Source: CAD feature listing. Evaluate the final solid. Frame: model axes, mm. A direction names the side the tool comes from. Coordinates: 2 decimals unless noted, no trailing zeros. Order: outer loops, then holes, each group sorted by start corner. A loop starts at its lowest first (then second) coordinate and runs counter-clockwise, first axis right, second up. Notation, with made-up numbers: (32.5, -33.5) - (78.5, -33.5) arc R25 cw to (78.5, -19.5) - close; hole circle Ø11 at (68.5, -31.5). An arc over 180 degrees is marked (long way). One line per question, with ' | ' between items. Start each with the question number.
(1) Line query: line 1 along Y through (x, z) = (3.5, 0.6); line 2 along X through (y, z) = (-6.75, 1.05); line 3 along Z through (x, y) = (18.25, -12.5). Output: solid intervals per line, ascending.
(2) Section A-A (z = 0.6). Return the cut outline in (x, y), then the cut area to 3 significant figures.
(3) Section B-B (y = -1.75). Return the cut outline in (x, z), then the cut area to 3 significant figures.
(4) Contact query for flat-ended pins moving along their axis: P1, Ø0.8, axis at x = 12.5, z = 1.5, coming from the -Y side; P2, Ø2.5, axis at x = 3.5, y = -2.1, coming from the +Z side; P3, Ø0.8, axis at x = 17, z = 1.5, coming from the +Y side. Output: stop coordinate, or through.
(5) Section D-D (y = -7.9). Return the cut outline in (x, z).
(6) Section C-C (x = 12.75). Return the cut outline in (y, z).
(7) Access query for faces 1 (the flat face through (14.035, -2, 1.5)), 2 (the flat face through (23.3, -0.5, 0.5)). Directions: +Z, -Z, +X, -X, +Y, -Y. A direction counts if a zero-diameter tool reaches every point of the face in a straight line with its end or side. Return the directions, or none.
(8) Draft query along Y for faces 3 (the cylindrical face through (22.5, -7.9, 0.5)), 4 (the cylindrical face through (22.5, -3.9, 0.5)), 5 (the flat face through (12, -2, 2)), 6 (the flat face through (11.8, -13.7, 0.5)). Return one class per face: +Y half, -Y half, draft (parallel to the pull), parting line (faces both ways), or undercut.
from build123d import *
from build123d.topology import SkipClean

# Parameters (mm, degrees)
SKETCH1_R           = 0.911145061
BOSS_EXTRUDE1_DEPTH = 1
SKETCH2_W           = 7.631466846
SKETCH2_H           = 13.7
BOSS_EXTRUDE2_DEPTH = 0.1
SKETCH3_W           = 5.617836281
SKETCH3_H           = 5.617836281
SKETCH3_W_2         = 4.333759416
SKETCH3_H_2         = 2.636943561
BOSS_EXTRUDE3_DEPTH = 2


with BuildPart() as part:
    # Sketch1 → Boss-Extrude1 (new body)
    with BuildSketch(Plane.XY):
        with BuildLine():
            Line((23.3, -2.7), (23.3, -3.1))
            ThreePointArc((23.3, -3.1), (22.5, -3.9), (23.3, -4.7))
            Line((23.3, -4.7), (23.3, -5.1))
            ThreePointArc((23.3, -5.1), (22.5, -5.9), (23.3, -6.7))
            Line((23.3, -6.7), (23.3, -7.1))
            ThreePointArc((23.3, -7.1), (22.5, -7.9), (23.3, -8.7))
            Line((23.3, -8.7), (23.3, -9.1))
            ThreePointArc((23.3, -9.1), (22.5, -9.9), (23.3, -10.7))
            Line((23.3, -10.7), (23.3, -11.1))
            ThreePointArc((23.3, -11.1), (22.5, -11.9), (23.3, -12.7))
            Line((23.3, -12.7), (23.3, -13.7))
            Line((23.3, -13.7), (0, -13.7))
            Line((0, -13.7), (0, 0))
            Line((0, 0), (23.3, 0))
            Line((23.3, 0), (23.3, -1.1))
            ThreePointArc((23.3, -1.1), (22.5, -1.9), (23.3, -2.7))
        make_face()
        with Locations((3.5, -2.1)):
            Circle(SKETCH1_R, mode=Mode.SUBTRACT)
    extrude(amount=BOSS_EXTRUDE1_DEPTH)

    # Sketch2 → Boss-Extrude2 (add)
    with SkipClean():  # the faces are left unmerged after this step: merging them gives an invalid solid
        with BuildSketch(Plane.XY.offset(1)):
            with Locations((3.815733423, -6.85)):
                Rectangle(SKETCH2_W, SKETCH2_H)
            with BuildLine():
                ThreePointArc((2.952848723, -2.828567637), (3.092783142, -1.284917334), (4.411145061, -2.1))
                ThreePointArc((4.411145061, -2.1), (3.907216858, -2.915082666), (2.952848723, -2.828567637))
            make_face(mode=Mode.SUBTRACT)
        extrude(amount=BOSS_EXTRUDE2_DEPTH)

    # Sketch3 → Boss-Extrude3 (add)
    with SkipClean():  # the faces are left unmerged after this step: merging them gives an invalid solid
        with BuildSketch(Plane.XY):
            with Locations((15.9493645, -8.202866697)):
                Rectangle(SKETCH3_W, SKETCH3_H)
            with Locations((11.867834468, -2.011781816)):
                Rectangle(SKETCH3_W_2, SKETCH3_H_2)
        extrude(amount=BOSS_EXTRUDE3_DEPTH)


solid = part.part
Response values:
1) line 1: y = -13.7 to -3.01, -1.19 to 0 | line 2: x = 0 to 7.63, 13.14 to 18.76 | line 3: z = 0 to 1
2) outline: (0, -13.7) - (23.3, -13.7) - (23.3, -12.7) arc R0.8 cw to (23.3, -11.1) - (23.3, -10.7) arc R0.8 cw to (23.3, -9.1) - (23.3, -8.7) arc R0.8 cw to (23.3, -7.1) - (23.3, -6.7) arc R0.8 cw to (23.3, -5.1) - (23.3, -4.7) arc R0.8 cw to (23.3, -3.1) - (23.3, -2.7) arc R0.8 cw to (23.3, -1.1) - (23.3, 0) - (0, 0) - close; hole circle Ø1.82 at (3.5, -2.1) | area: 311 mm²
3) outline: (0, 0) - (2.66, 0) - (2.66, 1.1) - (0, 1.1) - close; (4.34, 0) - (22.51, 0) - (22.51, 1) - (14.03, 1) - (14.03, 2) - (9.7, 2) - (9.7, 1) - (7.63, 1) - (7.63, 1.1) - (4.34, 1.1) - close | area: 25.8 mm²
4) P1: stops at y = -3.33 | P2: stops at z = 1.1 | P3: stops at y = -5.39
5) outline: (0, 0) - (22.5, 0) - (22.5, 1) - (18.76, 1) - (18.76, 2) - (13.14, 2) - (13.14, 1) - (7.63, 1) - (7.63, 1.1) - (0, 1.1) - close
6) outline: (-13.7, 0) - (0, 0) - (0, 1) - (-0.69, 1) - (-0.69, 2) - (-3.33, 2) - (-3.33, 1) - (-13.7, 1) - close
7) face 1: +Z, +X, +Y | face 2: +Z, -Z, +X, +Y, -Y
8) face 3: undercut | face 4: undercut | face 5: draft | face 6: -Y half
